Part model, mm, in its own coordinate system. A direction names the side the tool comes from. Coordinates: 2 decimals unless noted, no trailing zeros. Loops run counter-clockwise (first coordinate to the right, second up) from the corner with the lowest first, then second, coordinate; pieces in that order, holes last. Notation, with made-up numbers: (81.25, 48.5) -> (104.25, 48.5) arc R17 ccw to (104.25, 64.5) -> close; hole circle Ø11 at (32.25, 43). An arc over 180 degrees is marked (long way). Use one line per item in the form item = value. Start each with the question number.
(1) Band-saw the part on C-C on y = 5. Give the cut face in (x, z).
(2) Drill centre lines: L1, parallel to X at y = 22, z = 4.5; L2, parallel to X at y = 9, z = 6; L3, parallel to Y at x = -11, z = 22. Where is each one in solid material? Low to high. Write a range as [from, to].
(3) Band-saw the part on A-A on y = 10.5. Give the cut face in (x, z).
(4) 3-axis set-ups, long thin cutter, end or side, ignore diameter. For faces 4 (the flat face through (-4, 12.404, 20)), 5 (the flat face through (22, 16.404, 20)), 6 (the flat face through (-12.658, 21.2, 24.5)): which of +Z, -Z, +X, -X, +Y, -Y reach the whole face in a straight line?
(5) Pin check, flat tips, straight feed: P1, Ø4, axis at y = -3, z = 29.5, coming from the +X side; P2, Ø1, axis at x = -17, y = 13, coming from the +Z side; P3, Ø3, axis at y = 20.5, z = 24, coming from the +X side; P4, Ø2.5, axis at x = 13, z = 13, coming from the -Y side. Stop position of each tip, or through.
(6) Band-saw the part on B-B on x = 21. Give the cut face in (y, z).
(7) Mould opens along Z. For faces 1 (the flat face through (13.842, 10, 20)), 2 (the flat face through (0, 14, 40)), 3 (the flat face through (-11, 18.654, 20)) say: +Z half, -Z half, draft (parallel to the pull), parting line (faces both ways), or undercut.
```python
from build123d import *

# Parameters (mm, degrees)
F1_DEPTH = 40
F2_W     = 10.5
F2_H     = 17
F3_DEPTH = 4
F4_F1_R  = 1
F4_F2_R  = 1


with BuildPart() as f1:
    # F0 (on Top) → F1 (new body)
    with BuildSketch(Plane.XY):
        Polygon((-12.6578821212, 16.4037507206), (-21.6578821212, 16.4037507206), (-21.6578821212, -18.9613338028), (-17.6578821212, -18.9613338028), (-17.6578821212, 12.4037507206), (9.8421178788, 12.4037507206), (9.8421178788, 8.4037507206), (13.8421178788, 8.4037507206), (13.8421178788, 12.4037507206), (20.3421178788, 12.4037507206), (20.3421178788, 8.4037507206), (24.3421178788, 8.4037507206), (24.3421178788, 16.4037507206), (20.3421178788, 16.4037507206), (20.3421178788, 26.9037507206), (16.3421178788, 26.9037507206), (15.5421178788, 25.6037507206), (16.3421178788, 25.6037507206), (16.3421178788, 16.4037507206), (-8.6578821212, 16.4037507206), (-8.6578821212, 18.6537507206), (-12.6578821212, 18.6537507206), align=None)
    extrude(amount=F1_DEPTH)

    # F2 (on face) → F3 (join, through all)
    with BuildSketch(Plane(origin=(-12.6578821212, 0, 0), x_dir=(0, -1, 0), z_dir=(-1, 0, 0))):
        with Locations((-21.6537507206, 8.5)):
            Rectangle(F2_W, F2_H)
        with Locations((-21.6537507206, 31.5)):
            Rectangle(F2_W, F2_H)
    extrude(amount=-F3_DEPTH)

    # F4: fillet of radius 1 on 53 edges, made by hand

    # F4_f1
    f4_f1_edges = [f1.edges().sort_by_distance(p)[0] for p in [
        (-10.6578821212, 18.6537507206, 17),
        (-10.6578821212, 18.6537507206, 23),
        (-17.6578821212, 12.4037507206, 20),
    ]]
    fillet(f4_f1_edges, radius=F4_F1_R)

    # F4_f2
    f4_f2_edges = [f1.edges().sort_by_distance(p)[0] for p in [
        (20.3421178788, 26.9037507206, 20),
        (-10.6578821212, 26.9037507206, 17),
        (-10.6578821212, 26.9037507206, 23),
        (-10.6578821212, 26.9037507206, 0),
        (-10.6578821212, 26.9037507206, 40),
        (24.3421178788, 8.4037507206, 20),
        (9.8421178788, 8.4037507206, 20),
        (-21.6578821212, -18.9613338028, 20),
        (-12.6578821212, 21.6537507206, 40),
        (-12.6578821212, 21.6537507206, 0),
        (-12.6578821212, 26.9037507206, 8.5),
        (-12.6578821212, 26.9037507206, 31.5),
        (-17.1578821212, 16.4037507206, 0),
        (-17.1578821212, 16.4037507206, 40),
        (-21.6578821212, -1.2787915411, 40),
        (-21.6578821212, -1.2787915411, 0),
        (-19.6578821212, -18.9613338028, 40),
        (-19.6578821212, -18.9613338028, 0),
        (18.3421178788, 26.9037507206, 0),
        (18.3421178788, 26.9037507206, 40),
        (20.3421178788, 21.6537507206, 0),
        (20.3421178788, 21.6537507206, 40),
        (3.8421178788, 16.4037507206, 0),
        (3.8421178788, 16.4037507206, 40),
        (-3.4078821212, 12.4037507206, 0),
        (-3.4078821212, 12.4037507206, 40),
        (-17.6578821212, -18.9613338028, 20),
        (-8.6578821212, 21.6537507206, 0),
        (-8.6578821212, 26.9037507206, 8.5),
        (-8.6578821212, 26.9037507206, 31.5),
        (-8.6578821212, 21.6537507206, 40),
        (-12.6578821212, 23.2787507206, 17),
        (-8.6578821212, 23.2787507206, 17),
        (-8.6578821212, 18.6537507206, 20),
        (-12.6578821212, 18.6537507206, 20),
        (-12.6578821212, 23.2787507206, 23),
        (-8.6578821212, 23.2787507206, 23),
        (22.3421178788, 16.4037507206, 0),
        (24.3421178788, 12.4037507206, 0),
        (22.3421178788, 8.4037507206, 0),
        (9.8421178788, 10.4037507206, 0),
        (11.8421178788, 8.4037507206, 0),
        (17.0921178788, 12.4037507206, 0),
        (24.3421178788, 12.4037507206, 40),
        (22.3421178788, 8.4037507206, 40),
        (11.8421178788, 8.4037507206, 40),
        (9.8421178788, 10.4037507206, 40),
        (22.3421178788, 16.4037507206, 40),
        (24.3421178788, 16.4037507206, 20),
        (-21.6578821212, 16.4037507206, 20),
        (-8.6578821212, 18.9466439394, 22.7071067812),
        (-12.6578821212, 18.9466439394, 22.7071067812),
        (-12.6578821212, 18.9466439394, 17.2928932188),
        (-8.6578821212, 18.9466439394, 17.2928932188),
        (-17.3649889024, 12.1108575018, 40),
        (-17.3649889024, 12.1108575018, 0),
    ]]
    fillet(f4_f2_edges, radius=F4_F2_R)

    # F5 (on face) → F6 (revolve)
    with BuildSketch(Plane(origin=(0, 16.4037507206, 0), x_dir=(-1, 0, 0), z_dir=(0, 1, 0))):
        with BuildLine():
            Line((2.1578821212, 20), (-1.8421178788, 20))
            ThreePointArc((-1.8421178788, 20), (0.1578821212, 18), (2.1578821212, 20))
        make_face()
    revolve(axis=Axis((-0.1578821212, 16.4037507206, 20), (-1, 0, 0)))


solid = f1.part
```
A:
q1.outline = (-21.66, 1) arc R1 ccw to (-20.66, 0) -> (-18.66, 0) arc R1 ccw to (-17.66, 1) -> (-17.66, 39) arc R1 ccw to (-18.66, 40) -> (-20.66, 40) arc R1 ccw to (-21.66, 39) -> close
q2.L1 = [-12.66, -8.66], [16.34, 20.34]
q2.L2 = [-21.66, -17.66], [9.93, 13.84], [20.34, 24.26]
q2.L3 = [12.4, 18.65]
q3.outline = (-21.66, 1) arc R1 ccw to (-20.66, 0) -> (-18.66, 0) arc R1 ccw to (-17.66, 1) -> (-17.66, 39) arc R1 ccw to (-18.66, 40) -> (-20.66, 40) arc R1 ccw to (-21.66, 39) -> close; (9.84, 1) arc R1 ccw to (10.84, 0) -> (13.84, 0) -> (13.84, 40) -> (10.84, 40) arc R1 ccw to (9.84, 39) -> close; (20.34, 0) -> (23.34, 0) arc R1 ccw to (24.34, 1) -> (24.34, 39) arc R1 ccw to (23.34, 40) -> (20.34, 40) -> close
q4.face_4 = +Z, -Z, -Y
q4.face_5 = +Z, -Z, +X, +Y
q4.face_6 = +Z, -Z, -X, +Y
q5.P1 = -17.66
q5.P2 = 40
q5.P3 = 20.34
q5.P4 = 8.4
q6.outline = (8.4, 1) arc R1 ccw to (9.4, 0) -> (15.4, 0) arc R1 ccw to (16.4, 1) -> (16.4, 39) arc R1 ccw to (15.4, 40) -> (9.4, 40) arc R1 ccw to (8.4, 39) -> close
q7.face_1 = draft
q7.face_2 = +Z half
q7.face_3 = undercut
